Model file for the job. Use its own axes, mm. Face numbers are marked on the shaded views. A direction names the side the tool comes from. Give positions to 0.01 mm unless a question says otherwise; leave off trailing zeros. Loops run counter-clockwise (first coordinate to the right, second up) from the corner with the lowest first, then second, coordinate; pieces in that order, holes last. Notation, with made-up numbers: M 83.25,-20 L 128.25,-20 A24 cw 128.25,12 Z; hole C -6.5,-2.75 d6. An arc over 180 degrees is marked long. Answer in a Markdown table with one row per item.
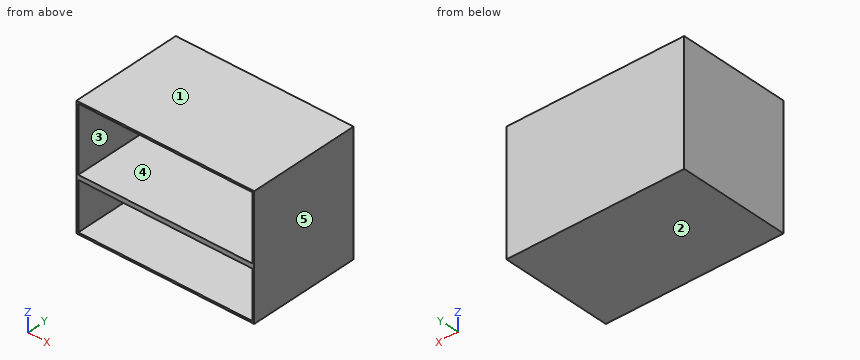
```python
from build123d import *

# Parameters (mm, degrees)
F0_W     = 241.3
F0_H     = 165.1
F1_DEPTH = 152.4
F2_T     = -2.54
F3_W     = 237.49
F3_H     = 152.4
F4_DEPTH = 6.35


with BuildPart() as f1:
    # F0 (on Front) → F1 (new body)
    with BuildSketch(Plane.XZ):
        with Locations((-4.36151, 14.835821)):
            Rectangle(F0_W, F0_H)
    extrude(amount=F1_DEPTH)

    # F2
    f2_openings = [f1.faces().sort_by_distance(p)[0] for p in [
        (-4.36151, -152.4, 14.835821),
    ]]
    offset(amount=F2_T, openings=f2_openings)

    # F3 (on Top) → F4 (join)
    with BuildSketch(Plane.XY):
        with Locations((-4.821002, -76.2)):
            Rectangle(F3_W, F3_H)
    extrude(amount=F4_DEPTH)


solid = f1.part
```
Q1. Mould opens along Z. For the marked faces 1, 2 and 3 say: released by +Z, released by -Z, zero draft, split by the parting line, or undercut.
Reported:
| item | result |
|---|---|
| face 1 | released by +Z |
| face 2 | released by -Z |
| face 3 | undercut |
Q2. Saw through at A-A (z = -56). Give the cut face in (x, y).
Reported:
| item | result |
|---|---|
| outline | M -125.01,-152.4 L -122.47,-152.4 L -122.47,-2.54 L 113.75,-2.54 L 113.75,-152.4 L 116.29,-152.4 L 116.29,0 L -125.01,0 Z |
Q3. Saw through at C-C (x = 74.5). Give the cut face in (y, z), and give its area (3 significant figures).
Reported:
| item | result |
|---|---|
| outline | M -152.4,-67.71 L 0,-67.71 L 0,97.39 L -152.4,97.39 L -152.4,94.85 L -2.54,94.85 L -2.54,6.35 L -152.4,6.35 L -152.4,0 L -2.54,0 L -2.54,-65.17 L -152.4,-65.17 Z |
| area | 2,130 mm² |
Q4. 3-axis set-ups, long thin cutter, end or side, ignore diameter. For the marked faces 4 and 5: which of +Z, -Z, +X, -X, +Y, -Y reach the whole face in a straight line?
Reported:
| item | result |
|---|---|
| face 4 | -Y |
| face 5 | +Z, -Z, +X, +Y, -Y |
Q5. Drop a flat-ended pin along its axis: pin 1 (1 mm diameter, centred on x = 50, z = 64, fed in from -Y). Give the stop position or say it passes through.
Reported:
| item | result |
|---|---|
| pin 1 | y = -2.54 |
Q6. Probe probe 1 along Z at (x, y) = (-65, -42.5); probe 2 along X at (y, z) = (-98, 75.5); probe 3 along Y at (x, z) = (-50, -52.5). List the from-to ranges inside material, lowest first.
Reported:
| item | result |
|---|---|
| probe 1 | -67.71 to -65.17, 0 to 6.35, 94.85 to 97.39 |
| probe 2 | -125.01 to -122.47, 113.75 to 116.29 |
| probe 3 | -2.54 to 0 |
Q7. Saw through at B-B (y = -107). Give the cut face in (x, z).
Reported:
| item | result |
|---|---|
| outline | M -125.01,-67.71 L 116.29,-67.71 L 116.29,97.39 L -125.01,97.39 Z; hole M -122.47,-65.17 L 113.75,-65.17 L 113.75,0 L -122.47,0 Z; hole M -122.47,6.35 L 113.75,6.35 L 113.75,94.85 L -122.47,94.85 Z |
